from build123d import *

# Parameters (mm, degrees)
SKETCH3_W          = 25
SKETCH3_H          = 2.5
CHAMFER1_SIZE      = 0.75
CUT_EXTRUDE1_DEPTH = 1.96
SKETCH9_R          = 1.732050808
CUT_EXTRUDE2_DEPTH = 1.96
CUT_EXTRUDE2_DRAFT = -45


with BuildPart() as part:
    # Sketch3 → Revolve1 (revolve)
    with BuildSketch(Plane(origin=(0, 0, 0), x_dir=(0, 0, -1), z_dir=(1, 0, 0))):
        with Locations((0, 1.25)):
            Rectangle(SKETCH3_W, SKETCH3_H)
    revolve(axis=Axis((0, 0, -12.5), (0, 0, 1)))

    # Chamfer1
    chamfer1_edges = [part.edges().sort_by_distance(p)[0] for p in [
        (0, -2.5, -12.5),
    ]]
    chamfer(chamfer1_edges, length=CHAMFER1_SIZE)

    # Sketch6 → Revolve2 (revolve)
    with BuildSketch(Plane(origin=(0, 0, 0), x_dir=(0, 0, -1), z_dir=(1, 0, 0))):
        Polygon((-12.5, 5), (-12.2, 5), (-9.7, 2.5), (-9.7, 0), (-12.5, 0), align=None)
    revolve(axis=Axis((0, 0, -12.5), (0, 0, 1)))

    # Sketch8 → Cut-Extrude1 (cut)
    with BuildSketch(Plane.XY.offset(12.5)):
        Polygon((0, 1.732050808), (-1.5, 0.866025404), (-1.5, -0.866025404), (0, -1.732050808), (1.5, -0.866025404), (1.5, 0.866025404), align=None)
    extrude(amount=-CUT_EXTRUDE1_DEPTH, mode=Mode.SUBTRACT)


with BuildPart() as cut_extrude2_tool:
    # Sketch9 → Cut-Extrude2 (with draft: the straight prism first)
    with BuildSketch(Plane.XY.offset(12.5)):
        Circle(SKETCH9_R)
    extrude(amount=-CUT_EXTRUDE2_DEPTH)
    # Cut-Extrude2: the draft: its side faces are tilted about the plane it starts from
    cut_extrude2_sides = [cut_extrude2_tool.faces().sort_by_distance(p)[0] for p in [
        (-1.732050808, 0, 11.52),
    ]]
    draft(cut_extrude2_sides, Plane.XY.offset(12.5), CUT_EXTRUDE2_DRAFT)


with BuildPart() as part_1:
    add(part.part)

    # Cut-Extrude2: cut by cut_extrude2_tool
    add(cut_extrude2_tool.part, mode=Mode.SUBTRACT)


solid = part_1.part
Source: CAD feature listing. Evaluate the final solid. Frame: model axes, mm. A direction names the side the tool comes from. Give positions to 0.01 mm unless a question says otherwise; leave off trailing zeros. Loops run counter-clockwise (first coordinate to the right, second up) from the corner with the lowest first, then second, coordinate; pieces in that order, holes last. Notation, with made-up numbers: (-20.75, 56.25) -> (32.25, 56.25) arc R23 cw to (32.25, 67.25) -> close; hole circle Ø7 at (5, 11.5). An arc over 180 degrees is marked (long way). Use a Markdown table: item, result. Add a question column.
1) Section query B-B, the plane z = -2.25. Return the cut outline in (x, y).
2) Section query A-A, the plane y = 0. Return the cut outline in (x, z).
3) Pull-direction query (X, two-part tool) for faces 3 (the face through (2.44, -0.54, -1.18)), 4 (the face through (0, 0, -12.5)), 5 (the face through (1.5, 0, 12)), 6 (the face through (0.819, 1.395, 12.386)); classes: +X half, -X half, draft (parallel to the pull), parting line (faces both ways), or undercut.
4) Line query: line 1 along Y through (x, z) = (2, 6.5); line 2 along Y through (x, z) = (1.25, 10); line 3 along Z through (x, y) = (0.25, 1). Output: solid intervals per line, ascending. Write a range as [from, to].
5) Reachability of faces 1 (the face through (4.88, -1.08, 12.35)), 2 (the face through (-1.5, 0, 12)) from +Z, -Z, +X, -X, +Y, -Y: full face, straight path, thin tool, end or side. Return the list, or none.
6) First-contact query: pin 1 (6 mm diameter, centred on x = 2.5, z = -3.5, fed in from +Y); pin 2 (1.4 mm diameter, centred on y = 0, z = 12, fed in from -X); pin 3 (1 mm diameter, centred on y = 0, z = 8, fed in from +X); pin 4 (2 mm diameter, centred on y = 2, z = 1, fed in from -X). Flat tips, straight axial feed; report the tip coordinate or a pass-through.
Numbers:
| question | item | result |
|---|---|---|
| 1 | outline | circle Ø5 at (0, 0) |
| 2 | outline | (-5, 12.2) -> (-2.5, 9.7) -> (-2.5, -11.75) -> (-1.75, -12.5) -> (1.75, -12.5) -> (2.5, -11.75) -> (2.5, 9.7) -> (5, 12.2) -> (5, 12.5) -> (1.73, 12.5) -> (1.5, 12.27) -> (1.5, 10.54) -> (-1.5, 10.54) -> (-1.5, 12.27) -> (-1.73, 12.5) -> (-5, 12.5) -> close |
| 3 | face 3 | parting line |
| 3 | face 4 | draft |
| 3 | face 5 | undercut |
| 3 | face 6 | undercut |
| 4 | line 1 | y = [-1.5, 1.5] |
| 4 | line 2 | y = [-2.51, 2.51] |
| 4 | line 3 | z = [-12.5, 10.54] |
| 5 | face 1 | +Z, -Z |
| 5 | face 2 | +Z |
| 6 | pin 1 | stops at y = 2.5 |
| 6 | pin 2 | stops at x = -5 |
| 6 | pin 3 | stops at x = 2.5 |
| 6 | pin 4 | stops at x = -2.29 |
